Part model, mm, in its own coordinate system. Face numbers are marked on the shaded views. A direction names the side the tool comes from. Round coordinates to 2 decimals unless told otherwise and drop trailing zeros. Loops run counter-clockwise (first coordinate to the right, second up) from the corner with the lowest first, then second, coordinate; pieces in that order, holes last. Notation, with made-up numbers: (70, 35.25) - (114, 35.25) arc R21 ccw to (114, 66.25) - close; hole circle Ø3 at (14, 10.5). An arc over 180 degrees is marked (long way). Write each question's results on one line, items separated by ' | '. Start each with the question number.
(1) Cut at A-A, the plane z = -0.5. List the corners of the cut face in (x, y).
(2) Cut at B-B, the plane x = 4.5. List the corners of the cut face in (y, z).
(3) Tool access for the marked faces 5 and 6: list every direction of +Z, -Z, +X, -X, +Y, -Y with a clear straight run to the whole face (end or side of a thin tool).
(4) Mould opens along X. For the marked faces 1, 2, 3 and 4 say: released by +X, released by -X, zero draft, split by the parting line, or undercut.
(5) Drill centre lines: L1, parallel to Z at x = 0, y = -5; L2, parallel to X at y = -2.25, z = 22; L3, parallel to Z at x = -4.5, y = -1.7. Where is each one in solid material? Low to high.
(6) Flat gauge pins, fed straight in: P1, Ø4, axis at x = 0, z = 4.99, coming from the +Y side; P2, Ø5.5, axis at x = -18.55, z = 22.01, coming from the -Y side. Where does each tip first touch, or does it go through?
(7) Cut at D-D, the plane y = -2.25. Give the number of separate pieces and of enclosed holes in the cut face, then the cut area to 3 significant figures.
(8) Cut at C-C, the plane x = 18.55. List the corners of the cut face in (y, z).
from build123d import *

# Parameters (mm, degrees)
F0_W     = 60
F0_H     = 50
F0_R     = 1.75
F1_DEPTH = 7
F2_SIZE  = 5
F3_R     = 3.25
F4_DEPTH = 4
F5_R     = 3.25
F6_DEPTH = 4
F8_DEPTH = 7.001
F9_SIZE  = 2


with BuildPart() as f1:
    # F0 (on Front) → F1 (new body)
    with BuildSketch(Plane.XZ):
        with Locations((0, 16.7464785278)):
            Rectangle(F0_W, F0_H)
        with Locations((-4.5, 14.9913392961)):
            Circle(F0_R, mode=Mode.SUBTRACT)
        with Locations((0, 4.9913392961)):
            Circle(F0_R, mode=Mode.SUBTRACT)
        with Locations((4.5, 14.9913392961)):
            Circle(F0_R, mode=Mode.SUBTRACT)
        with Locations((-18.55, 22.0145061612)):
            Circle(F0_R, mode=Mode.SUBTRACT)
        with Locations((18.55, 22.0145061612)):
            Circle(F0_R, mode=Mode.SUBTRACT)
    extrude(amount=F1_DEPTH)

    # F2
    f2_edges = [f1.edges().sort_by_distance(p)[0] for p in [
        (-30, -3.5, -8.253521),
        (30, -3.5, -8.253521),
        (30, -3.5, 41.746479),
        (-30, -3.5, 41.746479),
    ]]
    chamfer(f2_edges, length=F2_SIZE)

    # F3 (on face) → F4 (cut)
    with BuildSketch(Plane(origin=(0, 0, 0), x_dir=(-1, 0, 0), z_dir=(0, 1, 0))):
        with Locations((-4.5, 14.9913392961)):
            Circle(F3_R)
        with Locations((4.5, 14.9913392961)):
            Circle(F3_R)
        with Locations((0, 4.9913392961)):
            Circle(F3_R)
    extrude(amount=-F4_DEPTH, mode=Mode.SUBTRACT)

    # F5 (on face) → F6 (cut)
    with BuildSketch(Plane.XZ.offset(7)):
        with Locations((-18.55, 22.0145061612)):
            Circle(F5_R)
        with Locations((18.55, 22.0145061612)):
            Circle(F5_R)
    extrude(amount=-F6_DEPTH, mode=Mode.SUBTRACT)

    # F7 (on face) → F8 (cut, through all)
    with BuildSketch(Plane.XZ.offset(7)):
        Polygon((20, 36.7464785278), (0, 36.7464785278), (-20, 36.7464785278), (-10, 26.7464785278), (0, 26.7464785278), (10, 26.7464785278), align=None)
        Polygon((25, -3.2535214722), (25, 16.7464785278), (15, 6.7464785278), (15, -3.2535214722), align=None)
        Polygon((-15, 6.7464785278), (-25, 16.7464785278), (-25, -3.2535214722), (-15, -3.2535214722), align=None)
    extrude(amount=-F8_DEPTH, mode=Mode.SUBTRACT)

    # F9
    f9_edges = [f1.edges().sort_by_distance(p)[0] for p in [
        (0, -7, 41.746479),
        (27.5, -7, 39.246479),
        (-27.5, -7, 39.246479),
        (30, -7, 16.746479),
        (27.5, -7, -5.753521),
        (0, -7, -8.253521),
        (-27.5, -7, -5.753521),
        (-30, -7, 16.746479),
    ]]
    chamfer(f9_edges, length=F9_SIZE)


solid = f1.part
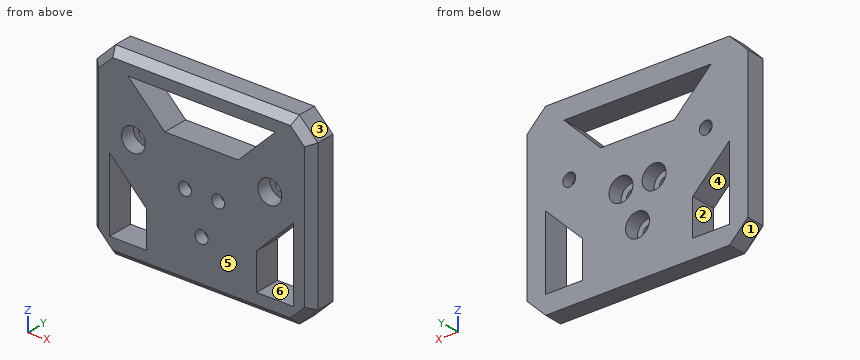
A:
1) outline: (-30, -5) - (-28, -7) - (-25, -7) - (-25, 0) - (-30, 0) - close; (-15, -7) - (15, -7) - (15, 0) - (-15, 0) - close; (25, -7) - (28, -7) - (30, -5) - (30, 0) - (25, 0) - close
2) outline: (-7, -6.25) - (-5, -8.25) - (0, -8.25) - (0, 11.74) - (-4, 11.74) - (-4, 13.24) - (-7, 13.24) - close; (-7, 16.74) - (-4, 16.74) - (-4, 18.24) - (0, 18.24) - (0, 26.75) - (-7, 26.75) - close; (-7, 36.75) - (0, 36.75) - (0, 41.75) - (-5, 41.75) - (-7, 39.75) - close
3) face 5: +Z, -Z, +X, -X, -Y | face 6: +Y, -Y
4) face 1: released by -X | face 2: undercut | face 3: released by +X | face 4: undercut
5) L1: -8.25 to 3.24, 6.74 to 26.75, 36.75 to 41.75 | L2: -30 to -20.3, -16.8 to 16.8, 20.3 to 30 | L3: -8.25 to 11.74, 18.24 to 26.75, 36.75 to 41.75
6) P1: y = -4 | P2: y = -3
7) separate pieces: 1 | enclosed holes: 8 | area: 2,230 mm2
8) outline: (-7, -6.25) - (-5, -8.25) - (0, -8.25) - (0, -3.25) - (-7, -3.25) - close; (-7, 10.3) - (0, 10.3) - (0, 20.26) - (-3, 20.26) - (-3, 18.76) - (-7, 18.76) - close; (-7, 25.26) - (-3, 25.26) - (-3, 23.76) - (0, 23.76) - (0, 35.3) - (-7, 35.3) - close; (-7, 36.75) - (0, 36.75) - (0, 41.75) - (-5, 41.75) - (-7, 39.75) - close
